Design review of the part built by this model. Coordinates are the model's own, in mm. A direction names the side the tool comes from. Give positions to 0.01 mm unless a question says otherwise; leave off trailing zeros. Order: outer loops, then holes, each group sorted by start corner. A loop starts at its lowest first (then second) coordinate and runs counter-clockwise, first axis right, second up.
```python
from build123d import *

# Parameters (mm, degrees)
SKETCH1_R           = 1.1
SKETCH1_R_2         = 1.55
BOSS_EXTRUDE1_DEPTH = 3.048


with BuildPart() as part:
    # Sketch1 → Boss-Extrude1 (new body)
    with BuildSketch(Plane(origin=(0, 0, 0), x_dir=(1, 0, 0), z_dir=(0, 1, 0))):
        with BuildLine():
            Line((-40.209744398, 44.711958299), (28.240255602, 44.711958299))
            ThreePointArc((28.240255602, 44.711958299), (44.41885963, 38.010560578), (51.120255602, 21.831955824))
            Line((51.120255602, 21.831955824), (51.120255602, -34.598189146))
            ThreePointArc((51.120255602, -34.598189146), (47.776738906, -42.160841434), (40.130306185, -45.308043388))
            Line((40.130306185, -45.308043388), (-40.209744398, -45.308043388))
            ThreePointArc((-40.209744398, -45.308043388), (-47.987919588, -42.086217385), (-51.209744398, -34.308041701))
            Line((-51.209744398, -34.308041701), (-51.209744398, 33.711958299))
            ThreePointArc((-51.209744398, 33.711958299), (-47.987918991, 41.490132892), (-40.209744398, 44.711958299))
        make_face()
        with Locations(Location((-39.019744398, -34.478043388, 0), (0, 0, 90))):
            Circle(SKETCH1_R, mode=Mode.SUBTRACT)
        with Locations(Location((-18.179744398, -34.478043388, 0), (0, 0, 90))):
            Circle(SKETCH1_R, mode=Mode.SUBTRACT)
        with Locations(Location((-39.019744398, 33.731958299, 0), (0, 0, 90))):
            Circle(SKETCH1_R, mode=Mode.SUBTRACT)
        with Locations(Location((8.610255602, 33.731915189, 0), (0, 0, 90))):
            Circle(SKETCH1_R, mode=Mode.SUBTRACT)
        with Locations(Location((8.655, 10.511958299, 0), (0, 0, 90))):
            Circle(SKETCH1_R, mode=Mode.SUBTRACT)
        with Locations(Location((-45.866598648, 39.368812549, 0), (0, 0, 90))):
            Circle(SKETCH1_R_2, mode=Mode.SUBTRACT)
        with Locations(Location((42.297539172, 35.889240349, 0), (0, 0, 90))):
            Circle(SKETCH1_R_2, mode=Mode.SUBTRACT)
        with Locations(Location((45.695011225, -40.000653974, 0), (0, 0, 90))):
            Circle(SKETCH1_R_2, mode=Mode.SUBTRACT)
        with Locations(Location((-45.858259021, -39.973270185, 0), (0, 0, 90))):
            Circle(SKETCH1_R_2, mode=Mode.SUBTRACT)
        with BuildLine():
            Line((-34.699744398, 24.391958299), (-6.394744398, 24.391958299))
            ThreePointArc((-6.394744398, 24.391958299), (-5.496718786, 24.019983911), (-5.124744398, 23.121958299))
            Line((-5.124744398, 23.121958299), (-5.124744398, 22.561958299))
            ThreePointArc((-5.124744398, 22.561958299), (-5.496718786, 21.663932687), (-6.394744398, 21.291958299))
            Line((-6.394744398, 21.291958299), (-34.699744398, 21.291958299))
            ThreePointArc((-34.699744398, 21.291958299), (-35.59777001, 21.663932687), (-35.969744398, 22.561958299))
            Line((-35.969744398, 22.561958299), (-35.969744398, 23.121958299))
            ThreePointArc((-35.969744398, 23.121958299), (-35.59777001, 24.019983911), (-34.699744398, 24.391958299))
        make_face(mode=Mode.SUBTRACT)
        with BuildLine():
            Line((35.880255602, 23.121958299), (35.880255602, 22.561958299))
            ThreePointArc((35.880255602, 22.561958299), (35.508281214, 21.663932687), (34.610255602, 21.291958299))
            Line((34.610255602, 21.291958299), (6.305255602, 21.291958299))
            ThreePointArc((6.305255602, 21.291958299), (5.40722999, 21.663932687), (5.035255602, 22.561958299))
            Line((5.035255602, 22.561958299), (5.035255602, 23.121958299))
            ThreePointArc((5.035255602, 23.121958299), (5.40722999, 24.019983911), (6.305255602, 24.391958299))
            Line((6.305255602, 24.391958299), (34.610255602, 24.391958299))
            ThreePointArc((34.610255602, 24.391958299), (35.508281214, 24.019983911), (35.880255602, 23.121958299))
        make_face(mode=Mode.SUBTRACT)
        with BuildLine():
            Line((35.880255602, -23.718041701), (35.880255602, -23.158041701))
            ThreePointArc((35.880255602, -23.158041701), (35.508281214, -22.260016089), (34.610255602, -21.888041701))
            Line((34.610255602, -21.888041701), (6.305255602, -21.888041701))
            ThreePointArc((6.305255602, -21.888041701), (5.40722999, -22.260016089), (5.035255602, -23.158041701))
            Line((5.035255602, -23.158041701), (5.035255602, -23.718041701))
            ThreePointArc((5.035255602, -23.718041701), (5.40722999, -24.616067313), (6.305255602, -24.988041701))
            Line((6.305255602, -24.988041701), (34.610255602, -24.988041701))
            ThreePointArc((34.610255602, -24.988041701), (35.508281214, -24.616067313), (35.880255602, -23.718041701))
        make_face(mode=Mode.SUBTRACT)
        with BuildLine():
            Line((-5.124744398, -23.718041701), (-5.124744398, -23.158041701))
            ThreePointArc((-5.124744398, -23.158041701), (-5.496718786, -22.260016089), (-6.394744398, -21.888041701))
            Line((-6.394744398, -21.888041701), (-34.699744398, -21.888041701))
            ThreePointArc((-34.699744398, -21.888041701), (-35.59777001, -22.260016089), (-35.969744398, -23.158041701))
            Line((-35.969744398, -23.158041701), (-35.969744398, -23.718041701))
            ThreePointArc((-35.969744398, -23.718041701), (-35.59777001, -24.616067313), (-34.699744398, -24.988041701))
            Line((-34.699744398, -24.988041701), (-6.394744398, -24.988041701))
            ThreePointArc((-6.394744398, -24.988041701), (-5.496718786, -24.616067313), (-5.124744398, -23.718041701))
        make_face(mode=Mode.SUBTRACT)
    extrude(amount=BOSS_EXTRUDE1_DEPTH)


solid = part.part
```
1. For line 1 along Z through (x, y) = (-17, 2); line 2 along Z through (x, y) = (8.5, 1.2); line 3 along Z through (x, y) = (-39, 2.1), list the stretches that pass through material, from the lowest coordinate up.
Recorded:
line 1: z = -44.71 to -24.39, -21.29 to 21.89, 24.99 to 45.31
line 2: z = -44.71 to -34.83, -32.64 to -24.39, -21.29 to -11.6, -9.42 to 21.89, 24.99 to 45.31
line 3: z = -44.71 to -34.83, -32.63 to 33.38, 35.58 to 45.31
2. For pin 1 (4 mm diameter, centred on x = -2, z = -19.5, fed in from -Y), flat-tipped, find the tip position at first contact; note if it passes through.
Recorded:
pin 1: stops at y = 0
3. Machinability: for faces 5 (the face through (20, 2, -24.392)), 6 (the face through (44.24, 1.5, -38.19)), which of the approach directions +Z, -Z, +X, -X, +Y, -Y give a long, thin tool a straight path to every point of the face, cutting with its end or side? Answer none if there is none.
Recorded:
face 5: +Y, -Y
face 6: -Z, +X, +Y, -Y
4. Take a section at C-C (y = 2.1). State how many separate pieces and enclosed holes the cut face has, then the cut area to 4 significant figures.
Recorded:
separate pieces: 1
enclosed holes: 13
area: 8,595 mm2
5. Take a section at A-A (x = -21). State the section outline as (y, z) points, then the cut area to 3 significant figures.
Recorded:
outline: (0, -44.71) - (3.05, -44.71) - (3.05, -24.39) - (0, -24.39) - close; (0, -21.29) - (3.05, -21.29) - (3.05, 21.89) - (0, 21.89) - close; (0, 24.99) - (3.05, 24.99) - (3.05, 45.31) - (0, 45.31) - close
area: 255 mm2
6. Take a section at B-B (z = -39). State the section outline as (x, y) points.
Recorded:
outline: (-49.86, 0) - (-47.37, 0) - (-47.37, 3.05) - (-49.86, 3.05) - close; (-44.36, 0) - (43.36, 0) - (43.36, 3.05) - (-44.36, 3.05) - close
7. Draft analysis for pull direction Z (two halves, no side actions). For faces 1 (the face through (-20, 2, -21.292)), 2 (the face through (1, 3.048, 0)), 3 (the face through (-48.073, 1.503, -41.404)), 4 (the face through (1, 2, 45.308)), state which applies: pulls with the +Z half, pulls with the -Z half, needs draft (parallel to the pull), parting line crosses it, or undercut.
Recorded:
face 1: undercut
face 2: needs draft
face 3: pulls with the -Z half
face 4: pulls with the +Z half
8. Take a section at D-D (x = 38). State the section outline as (y, z) points, then the cut area to 3 significant figures.
Recorded:
outline: (0, -42.53) - (3.05, -42.53) - (3.05, 45.31) - (0, 45.31) - close
area: 268 mm2
